```python
from build123d import *

# Parameters (mm, degrees)
F0_R           = 38.1
F0_R_2         = 9.525
F1_DEPTH       = 12.7
F2_R           = 12.7
F3_DEPTH       = 6.35
F5_D           = 3.175
F5_CBORE_D     = 6.35
F5_CBORE_DEPTH = 6.35


with BuildPart() as f1:
    # F0 (on Front) → F1 (new body)
    with BuildSketch(Plane.XZ):
        with Locations((-20.073514, 16.948864)):
            Circle(F0_R)
        with Locations((-20.073514, 16.948864)):
            Circle(F0_R_2, mode=Mode.SUBTRACT)
    extrude(amount=F1_DEPTH)

    # F2 (on face) → F3 (cut)
    with BuildSketch(Plane.XZ.offset(12.7)):
        with Locations((-20.073514, 16.948864)):
            Circle(F2_R)
    extrude(amount=-F3_DEPTH, mode=Mode.SUBTRACT)

    # F5 (through all)
    with Locations(Plane.XZ.offset(12.7)):
        with Locations((-20.073514, 48.698864), (-51.823514, 16.948864), (-20.073514, -14.801136), (11.676486, 16.948864)):
            CounterBoreHole(F5_D / 2, F5_CBORE_D / 2, F5_CBORE_DEPTH)


solid = f1.part
```
Could you check a few things on this model? Use its own coordinates, in mm. A direction names the side the tool comes from. Round coordinates to 2 decimals unless told otherwise and drop trailing zeros. Order: outer loops, then holes, each group sorted by start corner. A loop starts at its lowest first (then second) coordinate and runs counter-clockwise, first axis right, second up. Notation, with made-up numbers: M 47.25,87 L 104.25,87 A19 cw 104.25,117 Z; hole C 62.5,37.5 d2. An arc over 180 degrees is marked long. One line per question, with ' | ' between items. Start each with the question number.
(1) For P1, Ø5, axis at x = -20, z = 49, coming from the -Y side; P2, Ø3, axis at x = -23.5, y = -5, coming from the -Z side; P3, Ø1.5, axis at x = 6, y = -2.5, coming from the -Z side, each with a flat end and sliding along its axis, tell me the tip position at first contact or that it passes through.
(2) Thinking about a two-plate mould opening in X: for faces 3 (the face through (-19, -6.35, -13)), 4 (the face through (-4, -12.7, 17)), 5 (the face through (15.121, -6.261, 2.356)), which applies, +X half, -X half, draft (parallel to the pull), parting line (faces both ways), or undercut?
(3) Suppose I cut it at D-D on x = -3. List the corners of the cut face in (y, z) for me, then the cut area to 3 significant figures.
(4) For faces 1 (the face through (-18.488, -3.131, -14.731)), 2 (the face through (-55, -10, 17)), which set-ups out of +Z, -Z, +X, -X, +Y, -Y let a thin tool reach every point of the face, with its end or its side?
(5) Suppose I cut it at A-A on z = 12. List the corners of the cut face in (x, y) for me.
(6) Please list where these lines run through material, in increasing order: line 1 along Z through (x, y) = (-18, -6); line 2 along Z through (x, y) = (11.5, -1); line 3 along X through (y, z) = (-4.75, 13.5).
(7) Suppose I cut it at C-C on z = 2. List the corners of the cut face in (x, y) for me.
(8) Suppose I cut it at B-B on y = -3. Count the separate pieces of the cut face and the enclosed holes in it, then the cut area to 3 significant figures.
Geometry results:
1) P1: y = -6.35 | P2: z = -21.1 | P3: z = -11.52
2) face 3: undercut | face 4: draft | face 5: parting line
3) outline: M -12.7,-17.11 L 0,-17.11 L 0,51.01 L -12.7,51.01 Z | area: 865 mm²
4) face 1: +Y, -Y | face 2: -Y
5) outline: M -57.85,-12.7 L -31.77,-12.7 L -31.77,-6.35 L -28.21,-6.35 L -28.21,0 L -57.85,0 Z; M -11.94,-6.35 L -8.38,-6.35 L -8.38,-12.7 L 17.7,-12.7 L 17.7,0 L -11.94,0 Z
6) line 1: -21.09 to 7.65, 26.25 to 54.99 | line 2: -4.38 to 15.37, 18.53 to 38.27 | line 3: -58.02 to -28.95, -11.19 to 17.87
7) outline: M -55.12,-12.7 L 14.97,-12.7 L 14.97,0 L -55.12,0 Z
8) separate pieces: 1 | enclosed holes: 5 | area: 4,240 mm²
